Model file for the job. Use its own axes, mm. A direction names the side the tool comes from. Round coordinates to 2 decimals unless told otherwise and drop trailing zeros. Loops run counter-clockwise (first coordinate to the right, second up) from the corner with the lowest first, then second, coordinate; pieces in that order, holes last. Notation, with made-up numbers: (-4, 21.25) - (54, 21.25) arc R21 cw to (54, 38.25) - close; hole circle Ø8 at (21, 44). An arc over 180 degrees is marked (long way). Use one line per item in the form item = value.
from build123d import *

# Parameters (mm, degrees)
SKETCH098_W       = 1
SKETCH098_H       = 1
PAD061_DEPTH      = 4
SKETCH099_R       = 3
PAD062_DEPTH      = 3
PAD062_DEPTH_BACK = 3
SKETCH102_R       = 1.7
PAD063_DEPTH      = 8
SKETCH100_W       = 2.25
SKETCH100_H       = 2.25
POCKET048_DEPTH   = 2.5


with BuildPart() as part:
    # Sketch098 → Pad061 (new body)
    with BuildSketch(Plane(origin=(0, 0, 22), x_dir=(1, 0, 0), z_dir=(0, 0, -1))):
        with Locations((5.5, 22.5)):
            Rectangle(SKETCH098_W, SKETCH098_H)
    extrude(amount=-PAD061_DEPTH)

    # Sketch099 (on Face5 of Pad061) → Pad062 (join, two sides)
    with BuildSketch(Plane(origin=(0, 0, 22), x_dir=(1, 0, 0), z_dir=(0, 0, -1))) as pad062_sk:
        with Locations((5.5, 22.5)):
            Circle(SKETCH099_R)
    extrude(amount=PAD062_DEPTH)
    extrude(pad062_sk.sketch, amount=-PAD062_DEPTH_BACK)

    # Sketch102 → Pad063 (join)
    with BuildSketch(Plane.XY.offset(22)):
        with Locations((5.5, -22.5)):
            Circle(SKETCH102_R)
    extrude(amount=PAD063_DEPTH)

    # Sketch100 (on Face4 of Pad063) → Pocket048 (cut)
    with BuildSketch(Plane(origin=(0, 0, 19), x_dir=(1, 0, 0), z_dir=(0, 0, -1))):
        with Locations((5.5, 22.5)):
            Rectangle(SKETCH100_W, SKETCH100_H)
    extrude(amount=-POCKET048_DEPTH, mode=Mode.SUBTRACT)


solid = part.part
1. Flat gauge pins, fed straight in: pin 1 (2 mm diameter, centred on y = -21, z = 22, fed in from +X); pin 2 (2 mm diameter, centred on x = 7.5, z = 27.5, fed in from -Y); pin 3 (1.8 mm diameter, centred on x = 5.5, y = -22.5, fed in from -Z). Where does each tip first touch, or does it go through?
Geometry check:
pin_1 = 8.46
pin_2 = -23.87
pin_3 = 21.5
2. Tool access for faces 4 (the flat face through (7, -21, 25)), 5 (the flat face through (5, -21.375, 20)), 6 (the flat face through (5, -21, 19)): list every direction of +Z, -Z, +X, -X, +Y, -Y with a clear straight run to the whole face (end or side of a thin tool).
Geometry check:
face_4 = +Z
face_5 = -Z
face_6 = -Z, +X, -X, +Y, -Y
3. Pull direction Y, two halves, no side cores. Call faces 1 (the flat face through (5, -22, 30)), 2 (the flat face through (5, -23.625, 20)), 3 (the cylindrical face through (8.27, -21.35, 21.96)): +Y half, -Y half, draft (parallel to the pull), parting line (faces both ways), or undercut.
Geometry check:
face_1 = draft
face_2 = undercut
face_3 = parting line
4. Cut at B-B, the plane y = -22.5. Give the cut face in (x, z) (3 decimals).
Geometry check:
outline = (2.5, 19) - (4.375, 19) - (4.375, 21.5) - (6.625, 21.5) - (6.625, 19) - (8.5, 19) - (8.5, 25) - (7.2, 25) - (7.2, 30) - (3.8, 30) - (3.8, 25) - (2.5, 25) - close
5. Cut at D-D, the plane z = 24.75. Give the cut face in (x, y), plus the area to 3 significant figures.
Geometry check:
outline = circle Ø6 at (5.5, -22.5)
area = 28.3 mm^2
6. Cut at C-C, the plane x = 5.5. Give the cut face in (y, z) (3 decimals).
Geometry check:
outline = (-25.5, 19) - (-23.625, 19) - (-23.625, 21.5) - (-21.375, 21.5) - (-21.375, 19) - (-19.5, 19) - (-19.5, 25) - (-20.8, 25) - (-20.8, 30) - (-24.2, 30) - (-24.2, 25) - (-25.5, 25) - close
7. Cut at A-A, the plane z = 20.5. Give the cut face in (x, y) (3 decimals).
Geometry check:
outline = circle Ø6 at (5.5, -22.5); hole (4.375, -23.625) - (6.625, -23.625) - (6.625, -21.375) - (4.375, -21.375) - close
8. Wall check: probe 1 along Y at (x, z) = (5.55, 20.5) (3 decimals); probe 2 along Z at (x, y) = (5.9, -20); probe 3 along Z at (x, y) = (5, -22.1). Give the ranges that are in metal, low to high.
Geometry check:
probe_1 = -25.5 to -23.625, -21.375 to -19.5
probe_2 = 19 to 25
probe_3 = 21.5 to 30
